Source: CAD feature listing. Evaluate the final solid. Frame: model axes, mm. A direction names the side the tool comes from. Round coordinates to 2 decimals unless told otherwise and drop trailing zeros. Loops run counter-clockwise (first coordinate to the right, second up) from the corner with the lowest first, then second, coordinate; pieces in that order, holes last. Notation, with made-up numbers: M 30.5,8.25 L 60.5,8.25 A32 ccw 60.5,41.25 Z; hole C -11.5,-9.5 d3. An arc over 180 degrees is marked long. Answer as CSV lines item,"result". Start each with the question number.
```python
from build123d import *

# Parameters (mm, degrees)
SKETCH1_W           = 150
SKETCH1_H           = 150
BOSS_EXTRUDE1_DEPTH = 10
SKETCH3_W           = 12
SKETCH3_H           = 12
CUT_EXTRUDE2_DEPTH  = 107.536378763
CUT_EXTRUDE1_DEPTH  = 107.536378763


with BuildPart() as part:
    # Sketch1 → Boss-Extrude1 (new body)
    with BuildSketch(Plane(origin=(0, 0, 0), x_dir=(1, 0, 0), z_dir=(0, 1, 0))):
        Rectangle(SKETCH1_W, SKETCH1_H)
    extrude(amount=BOSS_EXTRUDE1_DEPTH)

    # Sketch3 → Cut-Extrude2 (cut, through all)
    with BuildSketch(Plane(origin=(0, 10, 0), x_dir=(1, 0, 0), z_dir=(0, 1, 0))):
        Rectangle(SKETCH3_W, SKETCH3_H)
    extrude(amount=-CUT_EXTRUDE2_DEPTH, mode=Mode.SUBTRACT)

    # Sketch2 → Cut-Extrude1 (cut, through all)
    with BuildSketch(Plane(origin=(0, 10, 0), x_dir=(1, 0, 0), z_dir=(0, 1, 0))):
        with BuildLine():
            Line((20, 6), (55, 6))
            ThreePointArc((55, 6), (61, 0), (55, -6))
            Line((55, -6), (20, -6))
            ThreePointArc((20, -6), (14, 0), (20, 6))
        make_face()
    extrude(amount=-CUT_EXTRUDE1_DEPTH, mode=Mode.SUBTRACT)


solid = part.part
```
1) Section C-C, the plane z = 0. Return loops of the section in (x, y).
2) Section B-B, the plane y = 4.25. Return loops of the section in (x, z), and give its area (3 significant figures).
3) Access query for faces 1 (the flat face through (-18, 0, -1)), 2 (the flat face through (37, 5, -6)). Directions: +Z, -Z, +X, -X, +Y, -Y. A direction counts if a zero-diameter tool reaches every point of the face in a straight line with its end or side. Return the directions, or none.
4) Section A-A, the plane x = 27. Return loops of the section in (y, z), and give its area (3 significant figures).
5) Mould query, pull axis X, two halves, no side actions, for faces 3 (the flat face through (-1, 5, 75)), 4 (the flat face through (75, 5, 1)), 5 (the flat face through (38, 5, 6)). Classes: pulls with the +X half, pulls with the -X half, needs draft (parallel to the pull), parting line crosses it, or undercut.
6) Ray query, line 1 along Z through (x, y) = (42, 3.25); line 2 along X through (y, z) = (2.25, 5). Return the intervals inside material, ascending.
Findings below:
1,outline,"M -75,0 L -6,0 L -6,10 L -75,10 Z; M 6,0 L 14,0 L 14,10 L 6,10 Z; M 61,0 L 75,0 L 75,10 L 61,10 Z"
2,outline,"M -75,-75 L 75,-75 L 75,75 L -75,75 Z; hole M -6,-6 L 6,-6 L 6,6 L -6,6 Z; hole M 20,-6 L 55,-6 A6 ccw 55,6 L 20,6 A6 ccw Z"
2,area,"21,800 mm²"
3,face 1,"+Z, -Z, +X, -X, -Y"
3,face 2,"+Y, -Y"
4,outline,"M 0,-75 L 10,-75 L 10,-6 L 0,-6 Z; M 0,6 L 10,6 L 10,75 L 0,75 Z"
4,area,"1,380 mm²"
5,face 3,"needs draft"
5,face 4,"pulls with the +X half"
5,face 5,"undercut"
6,line 1,"-75 to -6, 6 to 75"
6,line 2,"-75 to -6, 6 to 16.68, 58.32 to 75"
